```python
from build123d import *

# Parameters (mm, degrees)
SKETCH1_R           = 8.5
BOSS_EXTRUDE1_DEPTH = 5
SKETCH2_R           = 10.5
BOSS_EXTRUDE2_DEPTH = 5
SKETCH3_R           = 5
CUT_EXTRUDE1_DEPTH  = 18.90251379
SKETCH4_R           = 6.5
CUT_EXTRUDE2_DEPTH  = 7
FILLET1_R           = 1
FILLET2_R           = 0.5


with BuildPart() as part:
    # Sketch1 → Boss-Extrude1 (new body)
    with BuildSketch(Plane(origin=(0, 0, 0), x_dir=(1, 0, 0), z_dir=(0, 1, 0))):
        with Locations(Location((0, 0, 0), (0, 0, 270))):
            Circle(SKETCH1_R)
    extrude(amount=BOSS_EXTRUDE1_DEPTH)

    # Sketch2 → Boss-Extrude2 (add)
    with BuildSketch(Plane(origin=(0, 5, 0), x_dir=(1, 0, 0), z_dir=(0, 1, 0))):
        with Locations(Location((0, 0, 0), (0, 0, 270))):
            Circle(SKETCH2_R)
    extrude(amount=BOSS_EXTRUDE2_DEPTH)

    # Sketch3 → Cut-Extrude1 (cut, through all)
    with BuildSketch(Plane(origin=(0, 10, 0), x_dir=(1, 0, 0), z_dir=(0, 1, 0))):
        with Locations(Location((0, 0, 0), (0, 0, 270))):
            Circle(SKETCH3_R)
    extrude(amount=-CUT_EXTRUDE1_DEPTH, mode=Mode.SUBTRACT)

    # Sketch4 → Cut-Extrude2 (cut)
    with BuildSketch(Plane(origin=(0, 10, 0), x_dir=(1, 0, 0), z_dir=(0, 1, 0))):
        with Locations(Location((0, 0, 0), (0, 0, 270))):
            Circle(SKETCH4_R)
    extrude(amount=-CUT_EXTRUDE2_DEPTH, mode=Mode.SUBTRACT)

    # Fillet1
    fillet1_edges = [part.edges().sort_by_distance(p)[0] for p in [
        (0, 10, -10.5),
    ]]
    fillet(fillet1_edges, radius=FILLET1_R)

    # Fillet2
    fillet2_edges = [part.edges().sort_by_distance(p)[0] for p in [
        (0, 10, -6.5),
    ]]
    fillet(fillet2_edges, radius=FILLET2_R)


solid = part.part
```
Geometry: final body of the model. Coordinates: model frame, mm. A direction names the side the tool comes from. Give positions to 0.01 mm unless a question says otherwise; leave off trailing zeros. Write each loop counter-clockwise with the first axis right and the second up, starting at its lowest first coordinate (ties: lowest second). Pieces come first, ordered by that corner, then holes.
1. Section query D-D, the plane y = 1.75. Return loops of the section in (x, z), then the cut area to 3 significant figures.
2. Reachability of faces 1 (the cylindrical face through (-4.88, 1.52, -1.08)), 2 (the flat face through (-5, 3, 2)) from +Z, -Z, +X, -X, +Y, -Y: full face, straight path, thin tool, end or side. Return the list, or none.
3. Section query B-B, the plane z = 0. Return loops of the section in (x, y).
4. Pin query (flat end, axial travel): P1, Ø1.5, axis at x = -2.5, y = 4, coming from the -Z side; P2, Ø1, axis at y = 8.5, z = -3.5, coming from the -X side; P3, Ø1.5, axis at x = 5, z = -2.5, coming from the +Y side. Return the tip coordinate at first contact, or that it passes through.
5. Draft query along X for faces 3 (the flat face through (0, 5, 9)), 4 (the cylindrical face through (-3.955, 6.296, -5.158)), 5 (the cylindrical face through (8.428, 2.465, -1.107)). Return one class per face: released by +X, released by -X, zero draft, split by the parting line, or undercut.
6. Section query C-C, the plane y = 7. Return loops of the section in (x, z), then the cut area to 3 significant figures.
7. Section query A-A, the plane x = 0. Return loops of the section in (y, z).
8. Line query: probe 1 along X at (y, z) = (1.9, 0); probe 2 along X at (y, z) = (7, 0); probe 3 along Y at (x, z) = (5, -7). Output: solid intervals per line, ascending.
Computed:
1. outline: circle Ø17 at (0, 0); hole circle Ø10 at (0, 0)
1. area: 148 mm2
2. face 1: +Y, -Y
2. face 2: +Y
3. outline: (-10.5, 5) - (-8.5, 5) - (-8.5, 0) - (-5, 0) - (-5, 3) - (-6.5, 3) - (-6.5, 9.5) arc R0.5 ccw to (-7, 10) - (-9.5, 10) arc R1 ccw to (-10.5, 9) - close; (5, 0) - (8.5, 0) - (8.5, 5) - (10.5, 5) - (10.5, 9) arc R1 ccw to (9.5, 10) - (7, 10) arc R0.5 ccw to (6.5, 9.5) - (6.5, 3) - (5, 3) - close
4. P1: stops at z = -8.32
4. P2: stops at x = -10.06
4. P3: stops at y = 3
5. face 3: zero draft
5. face 4: undercut
5. face 5: split by the parting line
6. outline: circle Ø21 at (0, 0); hole circle Ø13 at (0, 0)
6. area: 214 mm2
7. outline: (0, -8.5) - (5, -8.5) - (5, -10.5) - (9, -10.5) arc R1 ccw to (10, -9.5) - (10, -7) arc R0.5 ccw to (9.5, -6.5) - (3, -6.5) - (3, -5) - (0, -5) - close; (0, 5) - (3, 5) - (3, 6.5) - (9.5, 6.5) arc R0.5 ccw to (10, 7) - (10, 9.5) arc R1 ccw to (9, 10.5) - (5, 10.5) - (5, 8.5) - (0, 8.5) - close
8. probe 1: x = -8.5 to -5, 5 to 8.5
8. probe 2: x = -10.5 to -6.5, 6.5 to 10.5
8. probe 3: y = 5 to 10
